from build123d import *

# Parameters (mm, degrees)
SKETCH_1_R          = 31
EXTRUDE_1_DEPTH     = 15
SKETCH_2_R          = 21
EXTRUDE_2_DEPTH     = 10
SKETCH_3_R          = 12.5
CUT_EXTRUDE_1_DEPTH = 51.467811524
CUT_EXTRUDE_3_DEPTH = 51.467811524
CHAMFER_1_SIZE      = 2
CHAMFER_2_SIZE      = 2
CHAMFER_3_SIZE      = 2
CHAMFER_4_SIZE      = 2
CHAMFER_5_SIZE      = 2
FILLET_1_R          = 3


with BuildPart() as part:
    # 草图1 → 凸台-拉伸1 (new body)
    with BuildSketch(Plane.XY):
        Circle(SKETCH_1_R)
    extrude(amount=-EXTRUDE_1_DEPTH)

    # 草图2 → 凸台-拉伸2 (add)
    with BuildSketch(Plane(origin=(0, 0, -15), x_dir=(-1, 0, 0), z_dir=(0, 0, -1))):
        Circle(SKETCH_2_R)
    extrude(amount=EXTRUDE_2_DEPTH)

    # 草图3 → 切除-拉伸1 (cut, through all)
    with BuildSketch(Plane.XY):
        Circle(SKETCH_3_R)
    extrude(amount=-CUT_EXTRUDE_1_DEPTH, mode=Mode.SUBTRACT)

    # 草图4 → 切除-拉伸3 (cut, through all)
    with BuildSketch(Plane.XY):
        with BuildLine():
            Line((0, 15.8), (4, 15.8))
            Line((4, 15.8), (4, 11.842719282))
            ThreePointArc((4, 11.842719282), (0, 12.5), (-4, 11.842719282))
            Line((-4, 11.842719282), (-4, 15.8))
            Line((-4, 15.8), (0, 15.8))
        make_face()
    extrude(amount=-CUT_EXTRUDE_3_DEPTH, mode=Mode.SUBTRACT)

    # 倒角1
    chamfer_1_edges = [part.edges().sort_by_distance(p)[0] for p in [
        (-31, 0, 0),
    ]]
    chamfer(chamfer_1_edges, length=CHAMFER_1_SIZE)

    # 倒角2
    chamfer_2_edges = [part.edges().sort_by_distance(p)[0] for p in [
        (-31, 0, -15),
    ]]
    chamfer(chamfer_2_edges, length=CHAMFER_2_SIZE)

    # 倒角3
    chamfer_3_edges = [part.edges().sort_by_distance(p)[0] for p in [
        (0, -12.5, 0),
    ]]
    chamfer(chamfer_3_edges, length=CHAMFER_3_SIZE)

    # 倒角4
    chamfer_4_edges = [part.edges().sort_by_distance(p)[0] for p in [
        (0, -12.5, -25),
    ]]
    chamfer(chamfer_4_edges, length=CHAMFER_4_SIZE)

    # 倒角5
    chamfer_5_edges = [part.edges().sort_by_distance(p)[0] for p in [
        (21, 0, -25),
    ]]
    chamfer(chamfer_5_edges, length=CHAMFER_5_SIZE)

    # 圆角1
    fillet_1_edges = [part.edges().sort_by_distance(p)[0] for p in [
        (21, 0, -15),
    ]]
    fillet(fillet_1_edges, radius=FILLET_1_R)


solid = part.part
Geometry: final body of the model. Coordinates: model frame, mm. A direction names the side the tool comes from. Give positions to 0.01 mm unless a question says otherwise; leave off trailing zeros. Order: outer loops, then holes, each group sorted by start corner. A loop starts at its lowest first (then second) coordinate and runs counter-clockwise, first axis right, second up. Notation, with made-up numbers: (45.5, 61.25) -> (82.5, 61.25) arc R36 ccw to (82.5, 97.25) -> close; hole circle Ø3 at (65.25, 22). An arc over 180 degrees is marked (long way). Answer as a JSON object with one key per item and string values.
Q1. Section C-C (z = -9.25). Output: boundary loops of the cut face in (x, y).
Entries:
{"outline": "circle Ø62 at (0, 0); hole (-4, 11.84) arc R12.5 ccw (long way) to (4, 11.84) -> (4, 15.8) -> (-4, 15.8) -> close"}
Q2. First-contact query: pin 1 (10 mm diameter, centred on x = 8.5, y = -10.5, fed in from -Z); pin 2 (3 mm diameter, centred on y = 14.5, z = -10, fed in from -X); pin 3 (1.2 mm diameter, centred on y = 14, z = -18.5, fed in from +X); pin 4 (2.5 mm diameter, centred on x = 1, z = -18, fed in from -Y). Flat tips, straight axial feed; report the tip coordinate or a pass-through.
Entries:
{"pin 1": "stops at z = -25", "pin 2": "stops at x = -28.14", "pin 3": "stops at x = 16.17", "pin 4": "stops at y = -21.25"}
Q3. Access query for faces 1 (the flat face through (-13, 7, 0)), 2 (the flat face through (-4, 14, -12)), 3 (the cylindrical face through (-20.03, 6.31, -20.46)). Directions: +Z, -Z, +X, -X, +Y, -Y. A direction counts if a zero-diameter tool reaches every point of the face in a straight line with its end or side. Return the directions, or none.
Entries:
{"face 1": "+Z, +X, -X, +Y, -Y", "face 2": "+Z, -Z", "face 3": "-Z"}
Q4. Section D-D (z = -16.75). Output: boundary loops of the cut face in (x, y), plus the area to 3 significant figures.
Entries:
{"outline": "circle Ø42.55 at (0, 0); hole (-4, 11.84) arc R12.5 ccw (long way) to (4, 11.84) -> (4, 15.8) -> (-4, 15.8) -> close", "area": "903 mm^2"}
Q5. Section B-B (y = 0). Output: boundary loops of the cut face in (x, z).
Entries:
{"outline": "(-31, -13) -> (-29, -15) -> (-24, -15) arc R3 cw to (-21, -18) -> (-21, -23) -> (-19, -25) -> (-14.5, -25) -> (-12.5, -23) -> (-12.5, -2) -> (-14.5, 0) -> (-29, 0) -> (-31, -2) -> close; (12.5, -23) -> (14.5, -25) -> (19, -25) -> (21, -23) -> (21, -18) arc R3 cw to (24, -15) -> (29, -15) -> (31, -13) -> (31, -2) -> (29, 0) -> (14.5, 0) -> (12.5, -2) -> close"}
Q6. Section A-A (x = 0). Output: boundary loops of the cut face in (y, z).
Entries:
{"outline": "(-31, -13) -> (-29, -15) -> (-24, -15) arc R3 cw to (-21, -18) -> (-21, -23) -> (-19, -25) -> (-14.5, -25) -> (-12.5, -23) -> (-12.5, -2) -> (-14.5, 0) -> (-29, 0) -> (-31, -2) -> close; (15.8, -25) -> (19, -25) -> (21, -23) -> (21, -18) arc R3 cw to (24, -15) -> (29, -15) -> (31, -13) -> (31, -2) -> (29, 0) -> (15.8, 0) -> close"}
Q7. Material intervals for probe 1 along Y at (x, z) = (0, -11.75); probe 2 along Y at (x, z) = (-24.5, -2), sorted ascending.
Entries:
{"probe 1": "y = -31 to -12.5, 15.8 to 31", "probe 2": "y = -18.99 to 18.99"}
Q8. Draft query along X for faces 4 (the flat face through (0, 15.8, -12)), 5 (the flat face through (-11, 22, -15)), 6 (the cylindrical face through (-4.036, 30.736, -7.423)). Return one class per face: released by +X, released by -X, zero draft, split by the parting line, or undercut.
Entries:
{"face 4": "undercut", "face 5": "zero draft", "face 6": "split by the parting line"}
